The listing builds one solid part. Answer for the finished solid, in the listing's coordinates (mm). Round coordinates to 2 decimals unless told otherwise and drop trailing zeros. Loops run counter-clockwise (first coordinate to the right, second up) from the corner with the lowest first, then second, coordinate; pieces in that order, holes last. Notation, with made-up numbers: (37.25, 54) - (55.25, 54) arc R15 ccw to (55.25, 60) - close; hole circle Ø4 at (-14.75, -14). An arc over 180 degrees is marked (long way). One line per item, written item: value.
```python
from build123d import *

# Parameters (mm, degrees)
SZKIC1_W = 125
SZKIC1_H = 5


with BuildPart() as part:
    # Szkic1 → Obrót1 (revolve)
    with BuildSketch(Plane.XY, mode=Mode.PRIVATE) as obr_t1_sk:
        with Locations((62.5, 2.5)):
            Rectangle(SZKIC1_W, SZKIC1_H)
    obr_t1 = revolve(obr_t1_sk.sketch.rotate(Axis((0, 0, 0), (1, 0, 0)), 90), axis=Axis((0, 0, 0), (1, 0, 0)))

    # Szkic2 → Obrót3 (revolve)
    with BuildSketch(Plane(origin=(125, 0, 0), x_dir=(0, 0, -1), z_dir=(1, 0, 0))):
        with BuildLine():
            Line((-7.5, 0), (7.5, 0))
            ThreePointArc((7.5, 0), (0, 7.5), (-7.5, 0))
        make_face()
    obr_t3 = revolve(axis=Axis((125, 0, 7.5), (0, 0, -1)))

    # Lustro1: Obrót1, Obrót3 across plane
    add(obr_t1.mirror(Plane(origin=(0, 0, 0), x_dir=(0, 0, 1), z_dir=(1, 0, 0))))
    add(obr_t3.mirror(Plane(origin=(0, 0, 0), x_dir=(0, 0, 1), z_dir=(1, 0, 0))))


solid = part.part
```
1) Each of these flat-tipped pins is pushed along its axis until it touches: pin 1 Ø3 at (x, y) = (103, 5.5) entering from -Z; pin 2 Ø6 at (x, z) = (102.5, 1.5) entering from +Y; pin 3 Ø5 at (x, z) = (-85.5, 5.5) entering from -Y. Where does it stop, or does it pass through?
Final values:
pin 1: z = -3
pin 2: y = 5
pin 3: y = -4
2) Consider L1, parallel to X at y = -6.5, z = -2.5; L2, parallel to X at y = 5.5, z = -3; L3, parallel to Z at x = 37, y = -0.25. Determine where each line is inside the solid, lowest interval first.
Final values:
L1: -127.78 to -122.22, 122.22 to 127.78
L2: -129.12 to -120.88, 120.88 to 129.12
L3: -4.99 to 4.99
3) A cutting plane is placed at B-B on x = -89. Give the vertices of the cut face in (y, z).
Final values:
outline: circle Ø10 at (0, 0)
4) A cutting plane is placed at A-A on z = 0. Give the vertices of the cut face in (x, y), and give its area (3 significant figures).
Final values:
outline: (-119.41, -5) - (119.41, -5) arc R7.5 ccw (long way) to (119.41, 5) - (-119.41, 5) arc R7.5 ccw (long way) to start
area: 2,720 mm2
